For this review, take the finished solid that the model builds, in its own axes (mm). A direction names the side the tool comes from. Round coordinates to 2 decimals unless told otherwise and drop trailing zeros. Loops run counter-clockwise (first coordinate to the right, second up) from the corner with the lowest first, then second, coordinate; pieces in that order, holes last. Notation, with made-up numbers: M 19.25,61.5 L 78.25,61.5 A29 ccw 78.25,99.5 Z; hole C 10.25,-8 d1. An arc over 180 degrees is marked long. One line per question, with ' | ' between items. Start each with the question number.
1) We need section D-D (y = 62). Give the boundary of the cut face in (x, z), and give its area (3 significant figures).
2) Mouldability with a two-part tool opening along Y and no side actions: class faces 1 (the face through (-1, -25.584, 14)), 2 (the face through (-50.777, 0, 14)), 3 (the face through (12.987, -97.403, 3.757)) as pulls with the +Y half, pulls with the -Y half, needs draft (parallel to the pull), parting line crosses it, or undercut.
3) For pin 1 Ø12 at (x, y) = (4, -44) entering from +Z; pin 2 Ø4 at (x, z) = (-18.5, 13.5) entering from -Y; pin 3 Ø8 at (x, z) = (5, 11.5) entering from -Y; pin 4 Ø10.5 at (x, z) = (-3.5, 15.5) entering from +Y, all flat-tipped, find the tip position at first contact; note any pin that passes through.
4) We need section C-C (x = -31). Give the boundary of the cut face in (y, z), and give its area (3 significant figures).
5) For faces 4 (the face through (13.076, 97.404, 3.757)), 5 (the face through (-1, 25, 14)), list the 3-axis set-ups (+Z, -Z, +X, -X, +Y, -Y) from which the entire face can be reached by the end or side of a thin tool; tool diameter is ignored.
6) For probe 1 along X at (y, z) = (6.5, 10.75); probe 2 along Y at (x, z) = (9, 10); probe 3 along Z at (x, y) = (22, 19), list the stretches that pass through material, from the lowest coordinate up. Write a range as from..to.
7) We need section B-B (z = 10.75). Give the boundary of the cut face in (x, y).
```python
from build123d import *

# Parameters (mm, degrees)
F0_W     = 101.6
F0_H     = 203.2
F1_DEPTH = 7.62
F3_DEPTH = 25.4
F4_W     = 100
F4_H     = 50
F5_DEPTH = 12.954


with BuildPart() as f1:
    # F0 (on Top) → F1 (new body)
    with BuildSketch(Plane.XY):
        Rectangle(F0_W, F0_H)
    extrude(amount=F1_DEPTH)

    # F2 (on Top) → F3 (cut)
    with BuildSketch(Plane.XY):
        with BuildLine():
            Line((-15.035691, -77.822713), (-14.988321, -81.421245))
            ThreePointArc((-14.988321, -81.421245), (-13.081192, -83.592345), (-11.008666, -81.578528))
            Line((-11.008666, -81.578528), (-11.048887, -77.843856))
            ThreePointArc((-11.048887, -77.843856), (-13.031485, -75.796128), (-15.035691, -77.822713))
        make_face()
        with BuildLine():
            ThreePointArc((-15.035691, -95.377287), (-13.031485, -97.403872), (-11.048887, -95.356144))
            Line((-11.048887, -95.356144), (-11.008666, -91.621472))
            ThreePointArc((-11.008666, -91.621472), (-13.081192, -89.607655), (-14.988321, -91.778755))
            Line((-14.988321, -91.778755), (-15.035691, -95.377287))
        make_face()
        with BuildLine():
            ThreePointArc((15.035691, -77.822713), (13.031485, -75.796128), (11.048887, -77.843856))
            Line((11.048887, -77.843856), (11.008666, -81.578528))
            ThreePointArc((11.008666, -81.578528), (13.081192, -83.592345), (14.988321, -81.421245))
            Line((14.988321, -81.421245), (15.035691, -77.822713))
        make_face()
        with BuildLine():
            Line((11.008666, -91.621472), (11.048887, -95.356144))
            ThreePointArc((11.048887, -95.356144), (13.031485, -97.403872), (15.035691, -95.377287))
            Line((15.035691, -95.377287), (14.988321, -91.778755))
            ThreePointArc((14.988321, -91.778755), (13.081192, -89.607655), (11.008666, -91.621472))
        make_face()
        with BuildLine():
            ThreePointArc((15.035691, 95.377287), (13.031485, 97.403872), (11.048887, 95.356144))
            Line((11.048887, 95.356144), (11.008666, 91.621472))
            ThreePointArc((11.008666, 91.621472), (13.081192, 89.607655), (14.988321, 91.778755))
            Line((14.988321, 91.778755), (15.035691, 95.377287))
        make_face()
        with BuildLine():
            Line((-11.008666, 91.621472), (-11.048887, 95.356144))
            ThreePointArc((-11.048887, 95.356144), (-13.031485, 97.403872), (-15.035691, 95.377287))
            Line((-15.035691, 95.377287), (-14.988321, 91.778755))
            ThreePointArc((-14.988321, 91.778755), (-13.081192, 89.607655), (-11.008666, 91.621472))
        make_face()
        with BuildLine():
            ThreePointArc((-15.035691, 77.822713), (-13.031485, 75.796128), (-11.048887, 77.843856))
            Line((-11.048887, 77.843856), (-11.008666, 81.578528))
            ThreePointArc((-11.008666, 81.578528), (-13.081192, 83.592345), (-14.988321, 81.421245))
            Line((-14.988321, 81.421245), (-15.035691, 77.822713))
        make_face()
        with BuildLine():
            ThreePointArc((11.048887, 77.843856), (13.031485, 75.796128), (15.035691, 77.822713))
            Line((15.035691, 77.822713), (14.988321, 81.421245))
            ThreePointArc((14.988321, 81.421245), (13.081192, 83.592345), (11.008666, 81.578528))
            Line((11.008666, 81.578528), (11.048887, 77.843856))
        make_face()
    extrude(amount=F3_DEPTH, mode=Mode.SUBTRACT)

    # F4 (on face) → F5 (join)
    with BuildSketch(Plane.XY.offset(7.62)):
        Polygon((50, 25.5842), (-50, 25.5842), (-50.777242, 25), (-50.777242, -25), (-50, -25.5842), (50, -25.5842), (50.762001, -25), (50.762001, 25), align=None)
        Rectangle(F4_W, F4_H, mode=Mode.SUBTRACT)
    extrude(amount=F5_DEPTH)


solid = f1.part
```
Answers below:
1) outline: M -50.8,0 L 50.8,0 L 50.8,7.62 L -50.8,7.62 Z | area: 774 mm^2
2) face 1: pulls with the -Y half | face 2: needs draft | face 3: undercut
3) pin 1: z = 7.62 | pin 2: y = -25.58 | pin 3: y = -101.6 | pin 4: y = 25.58
4) outline: M -101.6,0 L 101.6,0 L 101.6,7.62 L 25.58,7.62 L 25.58,20.57 L 25,20.57 L 25,7.62 L -25,7.62 L -25,20.57 L -25.58,20.57 L -25.58,7.62 L -101.6,7.62 Z | area: 1,560 mm^2
5) face 4: +Z, -Z | face 5: +Z
6) probe 1: -50.78..-50, 50..50.76 | probe 2: -25.58..-25, 25..25.58 | probe 3: 0..7.62
7) outline: M -50.78,-25 L -50,-25.58 L 50,-25.58 L 50.76,-25 L 50.76,25 L 50,25.58 L -50,25.58 L -50.78,25 Z; hole M -50,-25 L 50,-25 L 50,25 L -50,25 Z
